Check sheet for the modelled part. Datum: model origin and axes. Units: mm. A direction names the side the tool comes from. Give positions to 0.01 mm unless a question says otherwise; leave off trailing zeros. Write each loop counter-clockwise with the first axis right and the second up, starting at its lowest first coordinate (ties: lowest second). Pieces come first, ordered by that corner, then holes. Notation, with made-up numbers: (72, 16.25) -> (91, 16.25) arc R14 cw to (91, 39.25) -> close; hole circle Ø8 at (5, 10). An arc over 180 degrees is marked (long way). Answer as a JSON object with one key per item and string values.
from build123d import *

# Parameters (mm, degrees)
SKETCH1_R               = 10
BOSS_EXTRUDE1_DEPTH     = 10.9
SKETCH2_R               = 4.9
SKETCH2_W               = 3.595890226
SKETCH2_H               = 3.8
CUT_EXTRUDE1_DEPTH      = 10
CUT_EXTRUDE1_DEPTH_BACK = 10
CHAMFER1_SIZE           = 1
SCALE1_SCALE            = 0.75
SCALE2_SCALE            = 0.85
FILLET1_R               = 0.4
FILLET2_R               = 0.5


with BuildPart() as part:
    # Sketch1 → Boss-Extrude1 (new body)
    with BuildSketch(Plane(origin=(0, 0, 0), x_dir=(0, 1, 0), z_dir=(0, 0, 1))):
        Circle(SKETCH1_R)
    extrude(amount=BOSS_EXTRUDE1_DEPTH)

    # Sketch2 → Cut-Extrude1 (cut, two sides)
    with BuildSketch(Plane.XY.offset(10.9)) as cut_extrude1_sk:
        Circle(SKETCH2_R)
        with Locations((-5.518690803, 0)):
            Rectangle(SKETCH2_W, SKETCH2_H)
    extrude(amount=CUT_EXTRUDE1_DEPTH, mode=Mode.SUBTRACT)
    extrude(cut_extrude1_sk.sketch, amount=-CUT_EXTRUDE1_DEPTH_BACK, mode=Mode.SUBTRACT)

    # Chamfer1
    chamfer1_edges = [part.edges().sort_by_distance(p)[0] for p in [
        (4.9, 0, 10.9),
        (-5.916635916, 1.9, 10.9),
        (-5.916635916, -1.9, 10.9),
        (-7.316635916, 0, 10.9),
    ]]
    chamfer(chamfer1_edges, length=CHAMFER1_SIZE)


with BuildPart() as part_1:
    # Scale1: scaled about (0.237766223, 0, 5.261412395)
    add(part.part.scale(SCALE1_SCALE).moved(Location((0.059441556, 0, 1.315353099))))


with BuildPart() as part_2:
    # Scale2: scaled about (0.237766223, 0, 5.261412395)
    add(part_1.part.scale(SCALE2_SCALE).moved(Location((0.035664933, 0, 0.789211859))))

    # Fillet1
    fillet1_edges = [part_2.edges().sort_by_distance(p)[0] for p in [
        (0.086190256, -6.375, 8.856011993),
    ]]
    fillet(fillet1_edges, radius=FILLET1_R)

    # Fillet2
    fillet2_edges = [part_2.edges().sort_by_distance(p)[0] for p in [
        (0.086190256, -6.375, 1.907261993),
    ]]
    fillet(fillet2_edges, radius=FILLET2_R)


solid = part_2.part
1. Mould release check, pull along X, two halves, no side actions. Record for faces 3 (the face through (3.208, -0.12, 5.39)), 4 (the face through (3.38, -0.13, 8.39)), 5 (the face through (0, 0, 1.907)), 6 (the face through (6.31, -1.38, 5.39)): released by +X, released by -X, zero draft, split by the parting line, or undercut.
Determined:
{"face 3": "undercut", "face 4": "undercut", "face 5": "zero draft", "face 6": "split by the parting line"}
2. Sectioned sample at A-A, the plane y = 0. Enter the section's corners in (x, z).
Determined:
{"outline": "(-6.29, 2.41) arc R0.5 ccw to (-5.79, 1.91) -> (5.96, 1.91) arc R0.5 ccw to (6.46, 2.41) -> (6.46, 8.46) arc R0.4 ccw to (6.06, 8.86) -> (3.85, 8.86) -> (3.21, 8.22) -> (3.21, 2.48) -> (-4.58, 2.48) -> (-4.58, 8.22) -> (-5.22, 8.86) -> (-5.89, 8.86) arc R0.4 ccw to (-6.29, 8.46) -> close"}
3. Go/stop test with flat-tipped pins: P1, Ø1.4, axis at x = -4, z = 5.5, coming from the -Y side; P2, Ø1, axis at y = 1, z = 3.5, coming from the +X side; P3, Ø3, axis at x = -0.5, z = 6.5, coming from the +Y side (3 decimals); P4, Ø3, axis at x = 4, z = 6, coming from the +Y side. Record where each tip stops, or that it passes through.
Determined:
{"P1": "y = -5.4", "P2": "x = 6.44", "P3": "y = 6.375", "P4": "y = 5.9"}
4. Scan lines: L1, parallel to X at y = 0, z = 5.6; L2, parallel to Z at x = 0.25, y = 2.75; L3, parallel to Y at x = -0.25, z = 6.75. Record each from-to range of solid material in increasing order. Write a range as [from, to].
Determined:
{"L1": "[-6.29, -4.58], [3.21, 6.46]", "L2": "[1.91, 2.48]", "L3": "[-6.37, -3.11], [3.11, 6.37]"}
5. Access from +Z, -Z, +X, -X, +Y, -Y to the whole of each face (thin tool, end or side, straight path). Record for faces 1 (the face through (-4.578, 0, 5)), 2 (the face through (4, 0, 8.856)).
Determined:
{"face 1": "+Z", "face 2": "+Z, +X, -X, +Y, -Y"}
